Here's how the part is built. I have some questions about the finished solid (model axes, mm). A direction names the side the tool comes from. Round coordinates to 2 decimals unless told otherwise and drop trailing zeros. Write each loop counter-clockwise with the first axis right and the second up, starting at its lowest first coordinate (ties: lowest second). Pieces come first, ordered by that corner, then holes. Notation, with made-up numbers: (16, 36) - (65, 36) arc R15 cw to (65, 63) - close; hole circle Ø4 at (12, 20.5). An arc over 180 degrees is marked (long way). One line per item, written item: value. Start each with the question number.
Item 1: Imagine slicing it at B-B, the plane x = 16. Please give me the cut outline in (y, z).
Item 2: For faces 1 (the face through (18.06, -98.6, -291.44)), 2 (the face through (34, -99, -13)), 3 (the face through (29, -99, -96)), 4 (the face through (14, -99, -344)), which set-ups out of +Z, -Z, +X, -X, +Y, -Y let a thin tool reach every point of the face, with its end or its side?
Item 3: If I drill on line 1 (X direction, y = -51.5, z = -233.5); line 2 (Z direction, x = 4.5, y = -68); line 3 (X direction, y = -69, z = -100.5), over which ranges is the centre line in solid material (lowest first)?
Item 4: Imagine slicing it at D-D, the plane z = -47.5. Please give me the cut outline in (x, y).
Item 5: Thinking about a two-plate mould opening in Z: for faces 5 (the face through (27, -99, -95)), 6 (the face through (13, -99, -346)), 7 (the face through (18, -99, 0)), 8 (the face through (0, -99, -171)), which applies, released by +Z, released by -Z, zero draft, split by the parting line, or undercut?
Item 6: For P1, Ø1, axis at y = -44, z = -107.5, coming from the +X side; P2, Ø3, axis at y = -65.5, z = -145, coming from the +X side; P3, Ø4, axis at y = -126.5, z = -168, coming from the +X side, each with a flat end and sliding along its axis, tell me the tip position at first contact or that it passes through.
Item 7: Imagine slicing it at A-A, the plane z = -107.5. Please give me the cut outline in (x, y), then the cut area to 3 significant figures.
Item 8: Imagine slicing it at C-C, the plane z = -154. Please give me the cut outline in (x, y).
```python
from build123d import *

# Parameters (mm, degrees)
F1_DEPTH = 200
F2_R     = 2


with BuildPart() as f1:
    # F0 (on Front) → F1 (new body)
    with BuildSketch(Plane.XZ):
        Polygon((36, 0), (0, 0), (0, -346), (27, -346), (27, -316), (8.874961, -266.201865), (8.874961, -176.201865), (29, -120.908776), (29, -70.908776), (27, -70.908776), (27, -120.556122), (6.874961, -175.849212), (6.874961, -266.554519), (25, -316.352654), (25, -344), (2, -344), (2, -2), (34, -2), (34, -23), (36, -23), align=None)
    extrude(amount=F1_DEPTH)

    # F2
    f2_edges = [f1.edges().sort_by_distance(p)[0] for p in [
        (0, -100, 0),
        (36, -100, 0),
        (34, -100, -2),
        (2, -100, -2),
        (0, -100, -346),
        (2, -100, -344),
        (27, -100, -346),
        (25, -100, -344),
        (25, -100, -316.352654),
        (27, -100, -316),
        (8.874961, -100, -266.201865),
        (6.874961, -100, -266.554519),
        (6.874961, -100, -175.849212),
        (8.874961, -100, -176.201865),
        (29, -100, -120.908776),
        (27, -100, -120.556122),
    ]]
    fillet(f2_edges, radius=F2_R)


solid = f1.part
```
Values follow:
1. outline: (-200, -346) - (0, -346) - (0, -344) - (-200, -344) - close; (-200, -291.63) - (0, -291.63) - (0, -285.78) - (-200, -285.78) - close; (-200, -156.63) - (0, -156.63) - (0, -150.78) - (-200, -150.78) - close; (-200, -2) - (0, -2) - (0, 0) - (-200, 0) - close
2. face 1: +X, +Y, -Y
2. face 2: -Z, +Y, -Y
2. face 3: -Z, +X, +Y, -Y
2. face 4: +Y, -Y
3. line 1: x = 0 to 2, 6.87 to 8.87
3. line 2: z = -346 to -344, -2 to 0
3. line 3: x = 0 to 2, 27 to 29
4. outline: (0, -200) - (2, -200) - (2, 0) - (0, 0) - close
5. face 5: undercut
5. face 6: released by -Z
5. face 7: released by +Z
5. face 8: zero draft
6. P1: stops at x = 29
6. P2: stops at x = 20.78
6. P3: stops at x = 12.59
7. outline: (0, -200) - (2, -200) - (2, 0) - (0, 0) - close; (27, -200) - (29, -200) - (29, 0) - (27, 0) - close
7. area: 800 mm^2
8. outline: (0, -200) - (2, -200) - (2, 0) - (0, 0) - close; (14.83, -200) - (16.96, -200) - (16.96, 0) - (14.83, 0) - close
